Can you work these out from the drawing? Everything is in mm from the part's minimum corner. A direction names the side the tool comes from. Round coordinates to 2 decimals unless told otherwise and drop trailing zeros. Order: outer loops, then holes, each group sorted by start corner. A loop starts at its lowest first (then second) coordinate and runs counter-clockwise, first axis right, second up. Notation, with made-up numbers: M 25.25,-28 L 38.25,-28 A17 cw 38.25,-9 Z; hole C 24.5,-27.5 d7. An arc over 180 degrees is marked long. Write each question's results on one line, items separated by ' | '. Start each with the question number.
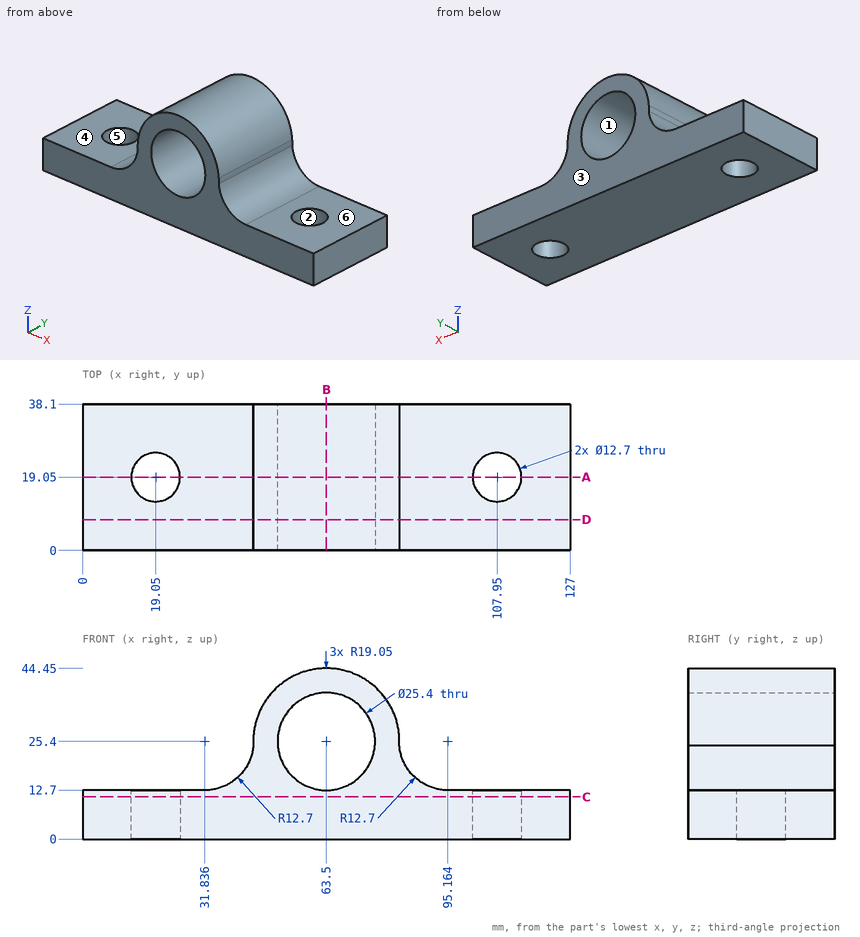
(1) I want a section at D-D on y = 8. Write out the boundary of the cut face in (x, z), and give its area (3 significant figures).
(2) I want a section at A-A on y = 19.05. Write out the boundary of the cut face in (x, z).
(3) I'm going to push flat-ended pins straight in: pin 1 Ø8 at (x, y) = (26.5, 30.5) entering from +Z; pin 2 Ø1 at (x, y) = (48, 16.5) entering from +Z; pin 3 Ø4 at (y, z) = (16.5, 39.5) entering from +X. Where does each tip first touch, or does it pass through?
(4) I want a section at B-B on x = 63.5. Write out the boundary of the cut face in (y, z).
(5) Please list where these lines run through material, in increasing order: line 1 (X direction, y = 19, z = 5); line 2 (Y direction, x = 19.05, z = 6.5); line 3 (Z direction, x = 63.5, y = 13).
(6) I want a section at C-C on z = 11. Write out the boundary of the cut face in (x, y).
(7) On a 3-axis mill with a long thin cutter (end or side, diameter ignored), from which of +Z, -Z, +X, -X, +Y, -Y can I reach the whole of each face in a straight line? I mean the marked faces 4, 5 and 6. Say none if no direction works.
(8) If we mould it in two halves opening along Y, with no side actions, what happens to the marked faces 1, 2 and 3? For each: pulls with the +Y half, pulls with the -Y half, needs draft (parallel to the pull), parting line crosses it, or undercut.
Solutions:
1) outline: M 0,0 L 127,0 L 127,12.7 L 95.16,12.7 A12.7 cw 82.52,24.26 A19.05 ccw 82.52,26.54 A19.05 ccw 44.48,26.54 A19.05 ccw 44.48,24.26 A12.7 cw 31.84,12.7 L 0,12.7 Z; hole C 63.5,25.4 d25.4 | area: 2,230 mm^2
2) outline: M 0,0 L 12.7,0 L 12.7,12.7 L 0,12.7 Z; M 25.4,0 L 101.6,0 L 101.6,12.7 L 95.16,12.7 A12.7 cw 82.52,24.26 A19.05 ccw 82.52,26.54 A19.05 ccw 44.48,26.54 A19.05 ccw 44.48,24.26 A12.7 cw 31.84,12.7 L 25.4,12.7 Z; M 114.3,0 L 127,0 L 127,12.7 L 114.3,12.7 Z; hole C 63.5,25.4 d25.4
3) pin 1: z = 12.7 | pin 2: z = 37.14 | pin 3: x = 78.21
4) outline: M 0,0 L 38.1,0 L 38.1,12.7 L 0,12.7 Z; M 0,38.1 L 38.1,38.1 L 38.1,44.45 L 0,44.45 Z
5) line 1: 0 to 12.7, 25.4 to 101.6, 114.3 to 127 | line 2: 0 to 12.7, 25.4 to 38.1 | line 3: 0 to 12.7, 38.1 to 44.45
6) outline: M 0,0 L 127,0 L 127,38.1 L 0,38.1 Z; hole C 19.05,19.05 d12.7; hole C 107.95,19.05 d12.7
7) face 4: +Z, -X, +Y, -Y | face 5: +Z, -Z | face 6: +Z, +X, +Y, -Y
8) face 1: needs draft | face 2: undercut | face 3: pulls with the +Y half
